from build123d import *

# Parameters (mm, degrees)
BOSS_EXTRUDE1_DEPTH = 6
SKETCH3_R           = 1.6
SKETCH3_W           = 222
SKETCH3_H           = 30.425305758
CUT_EXTRUDE1_DEPTH  = 10
SKETCH4_R           = 1.6
CUT_EXTRUDE2_DEPTH  = 10
CUT_EXTRUDE3_DEPTH  = 10


with BuildPart() as part:
    # Sketch1 → Boss-Extrude1 (new body)
    with BuildSketch(Plane(origin=(0, 0, 0), x_dir=(1, 0, 0), z_dir=(0, 1, 0))):
        Polygon((-111, 125.612652879), (111, 125.612652879), (111, -125.612652879), (111, -165.612652879), (-111, -165.612652879), (-111, -125.612652879), align=None)
    extrude(amount=BOSS_EXTRUDE1_DEPTH)

    # Sketch3 → Cut-Extrude1 (cut)
    with BuildSketch(Plane.XZ):
        with Locations(Location((66, 29.812652879, 0), (0, 0, 270))):
            Circle(SKETCH3_R)
        with Locations(Location((-66, 29.812652879, 0), (0, 0, 270))):
            Circle(SKETCH3_R)
        with Locations((0, -110.4)):
            Rectangle(SKETCH3_W, SKETCH3_H)
    extrude(amount=-CUT_EXTRUDE1_DEPTH, mode=Mode.SUBTRACT)

    # Sketch4 → Cut-Extrude2 (cut)
    with BuildSketch(Plane.XZ):
        with Locations(Location((87, 155.612652879, 0), (0, 0, 270))):
            Circle(SKETCH4_R)
        with Locations(Location((-87, 155.612652879, 0), (0, 0, 270))):
            Circle(SKETCH4_R)
        with Locations(Location((87, -85.187347121, 0), (0, 0, 270))):
            Circle(SKETCH4_R)
        with Locations(Location((-87, -85.187347121, 0), (0, 0, 270))):
            Circle(SKETCH4_R)
    extrude(amount=-CUT_EXTRUDE2_DEPTH, mode=Mode.SUBTRACT)

    # Sketch5 → Cut-Extrude3 (cut)
    with BuildSketch(Plane(origin=(0, 6, 0), x_dir=(1, 0, 0), z_dir=(0, 1, 0))):
        with BuildLine():
            Line((-50, -118.612652879), (50, -118.612652879))
            ThreePointArc((50, -118.612652879), (65, -133.612652879), (50, -148.612652879))
            Line((50, -148.612652879), (-50, -148.612652879))
            ThreePointArc((-50, -148.612652879), (-65, -133.612652879), (-50, -118.612652879))
        make_face()
    extrude(amount=-CUT_EXTRUDE3_DEPTH, mode=Mode.SUBTRACT)


solid = part.part
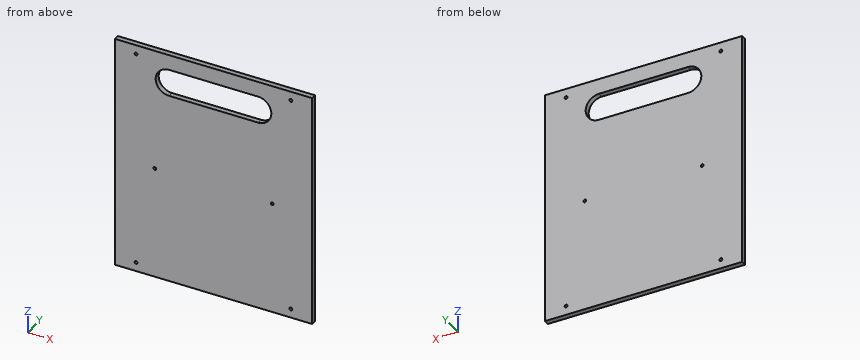
Here's how the part is built. I have some questions about the finished solid (model axes, mm). Coordinates: 2 decimals unless noted, no trailing zeros. Write each loop counter-clockwise with the first axis right and the second up, starting at its lowest first coordinate (ties: lowest second). Pieces come first, ordered by that corner, then holes.
Item 1: I want a section at A-A on x = -47. Write out the boundary of the cut face in (y, z).
Item 2: Will this pin go through, and if not, where does the flat tip stop? pin 1 (5 mm diameter, centred on x = 87, z = -85.19, fed in from -Y).
Item 3: I want a section at C-C on z = 137. Write out the boundary of the cut face in (x, y), and give its area (3 significant figures).
Item 4: I want a section at B-B on y = 2.15. Write out the boundary of the cut face in (x, z).
Item 5: If I drill on line 1 (Z direction, x = 87, y = 3.3); line 2 (Z direction, x = -1, y = 0.8); line 3 (Z direction, x = 66, y = 2.1), over which ranges is the centre line in solid material (lowest first)?
Findings below:
1. outline: (0, -95.19) - (6, -95.19) - (6, 118.61) - (0, 118.61) - close; (0, 148.61) - (6, 148.61) - (6, 165.61) - (0, 165.61) - close
2. pin 1: stops at y = 0
3. outline: (-111, 0) - (-64.61, 0) - (-64.61, 6) - (-111, 6) - close; (64.61, 0) - (111, 0) - (111, 6) - (64.61, 6) - close
3. area: 557 mm2
4. outline: (-111, -95.19) - (111, -95.19) - (111, 165.61) - (-111, 165.61) - close; hole circle Ø3.2 at (-87, -85.19); hole circle Ø3.2 at (-87, 155.61); hole circle Ø3.2 at (-66, 29.81); hole (-50, 118.61) - (50, 118.61) arc R15 ccw to (50, 148.61) - (-50, 148.61) arc R15 ccw to start; hole circle Ø3.2 at (66, 29.81); hole circle Ø3.2 at (87, -85.19); hole circle Ø3.2 at (87, 155.61)
5. line 1: z = -95.19 to -86.79, -83.59 to 154.01, 157.21 to 165.61
5. line 2: z = -95.19 to 118.61, 148.61 to 165.61
5. line 3: z = -95.19 to 28.21, 31.41 to 165.61
